Could you check a few things on this model? Use its own coordinates, in mm. Face numbers are marked on the shaded views. A direction names the side the tool comes from. Coordinates: 2 decimals unless noted, no trailing zeros. Order: outer loops, then holes, each group sorted by start corner. A loop starts at its lowest first (then second) coordinate and runs counter-clockwise, first axis right, second up. Notation, with made-up numbers: (-18, 33) -> (30, 33) arc R14 cw to (30, 54) -> close; hole circle Ø11 at (73, 75). An arc over 180 degrees is marked (long way). Use a Markdown table: item, result. Add a question column.
1) If I drill on L1, parallel to Z at x = 1.25, y = 1.45; L2, parallel to X at y = 0.6, z = 14; L3, parallel to X at y = -0.25, z = 15.5, over which ranges is the centre line in solid material (lowest first)? Write a range as [from, to].
2) If we section it at D-D (x = 2): Write out the boundary of the cut face in (y, z), plus the area to 3 significant figures.
3) Thinking about a two-plate mould opening in X: for the marked faces 1, 2 and 3, which applies, +X half, -X half, draft (parallel to the pull), parting line (faces both ways), or undercut?
4) If we section it at C-C (z = 14.5): Write out the boundary of the cut face in (x, y), plus the area to 3 significant figures.
5) If we section it at B-B (x = 0.8): Write out the boundary of the cut face in (y, z).
6) Will this pin go through, and if not, where does the flat tip stop? pin 1 Ø1.5 at (y, z) = (-1, 11.5) entering from +X.
7) If we section it at A-A (y = -0.85): Write out the boundary of the cut face in (x, z).
8) Which directions (+Z, -Z, +X, -X, +Y, -Y) give clear straight access to the entire face, cutting with the end or side of a thin tool? Please do the marked faces 4 and 5.
Autodesk Inventor part; units mm, degrees
ref_plane "YZ Plane" through (0, 0, 0) normal (1, 0, 0) x (0, 1, 0)
ref_plane "XZ Plane" through (0, 0, 0) normal (0, 1, 0) x (-1, 0, 0)
ref_plane "XY Plane" through (0, 0, 0) normal (0, 0, 1) x (1, 0, 0)
sketch "スケッチ1" plane through (0, 0, 0) normal (1, 0, 0) x (0, 1, 0)
  line L0 (0, 16.7) -> (0, 0)
  line L1 (0, 0) -> (2.4, 0)
  line L2 (2.4, 0) -> (2.4, 1.7)
  line L3 (2.4, 1.7) -> (1.3, 1.7)
  line L4 (1.3, 1.7) -> (1.3, 16.7)
  line L5 (1.3, 16.7) -> (0, 16.7)
  dimension "d2" = 1.7
  dimension "d10" = 15
  dimension "d11" = 2.6
  dimension "d12" = 4.8
revolve "回転1" add sketch "スケッチ1" angle 360 about axis through (0, 0, 16.7) along (0, 0, -1)
thread "ねじ1"
sketch "スケッチ2" plane through (0, 0, 0) normal (0, 0, -1) x (-1, 0, 0)
  line L0 (0, 1.1547) -> (1, 0.5774)
  line L1 (1, 0.5774) -> (1, -0.5774)
  line L2 (1, -0.5774) -> (0, -1.1547)
  line L3 (0, -1.1547) -> (-1, -0.5774)
  line L4 (-1, -0.5774) -> (-1, 0.5774)
  line L5 (-1, 0.5774) -> (0, 1.1547)
  line L6 (0, 2.4) -> (0, -2.4) construction
  circle A0 centre (0, 0) radius 2.4
  dimension "d7" = 2
extrude "押し出し1" cut sketch "スケッチ2" against normal blind 1.4 contours L0 L1 L2 L3 L4 L5
properties part number "M2_6-15" material "チタン"
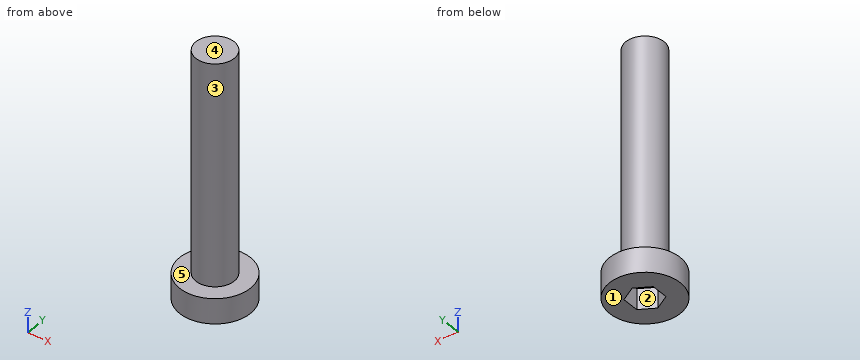
Answer sheet:
| question | item | result |
|---|---|---|
| 1 | L1 | [0, 1.7] |
| 1 | L2 | [-1.15, 1.15] |
| 1 | L3 | [-1.28, 1.28] |
| 2 | outline | (-1.33, 0) -> (1.33, 0) -> (1.33, 1.7) -> (-1.33, 1.7) -> close |
| 2 | area | 4.51 mm2 |
| 3 | face 1 | draft |
| 3 | face 2 | undercut |
| 3 | face 3 | parting line |
| 4 | outline | circle Ø2.6 at (0, 0) |
| 4 | area | 5.31 mm2 |
| 5 | outline | (-2.26, 0) -> (-0.69, 0) -> (-0.69, 1.4) -> (0.69, 1.4) -> (0.69, 0) -> (2.26, 0) -> (2.26, 1.7) -> (1.02, 1.7) -> (1.02, 16.7) -> (-1.02, 16.7) -> (-1.02, 1.7) -> (-2.26, 1.7) -> close |
| 6 | pin 1 | x = 1.28 |
| 7 | outline | (-2.24, 0) -> (-0.53, 0) -> (-0.53, 1.4) -> (0.53, 1.4) -> (0.53, 0) -> (2.24, 0) -> (2.24, 1.7) -> (0.98, 1.7) -> (0.98, 16.7) -> (-0.98, 16.7) -> (-0.98, 1.7) -> (-2.24, 1.7) -> close |
| 8 | face 4 | +Z, +X, -X, +Y, -Y |
| 8 | face 5 | +Z |
